Check sheet for the modelled part. Datum: model origin and axes. Units: mm. Face numbers are marked on the shaded views. A direction names the side the tool comes from. Coordinates: 2 decimals unless noted, no trailing zeros. Write each loop counter-clockwise with the first axis right and the second up, starting at its lowest first coordinate (ties: lowest second). Pieces come first, ordered by that corner, then holes. Notation, with made-up numbers: M 87,34 L 146,34 A22 ccw 146,40 Z; hole C -21,-19 d6. An arc over 180 degrees is marked long. Answer as CSV lines item,"result". Start each with the question number.
1) Section check C-C (y = 20.75). Record the cut outline in (x, z).
2) Section check A-A (y = 4.5). Record the cut outline in (x, z).
3) Go/stop test with flat-tipped pins: pin 1 Ø2 at (x, y) = (-15.5, 4) entering from -Z; pin 2 Ø6 at (y, z) = (7.5, 2.5) entering from +X; pin 3 Ø1 at (x, y) = (-15, 4.5) entering from +Z. Record where each tip stops, or that it passes through.
4) Section check D-D (x = -6). Record the cut outline in (y, z).
5) Section check B-B (z = -12). Record the cut outline in (x, y).
6) Access from +Z, -Z, +X, -X, +Y, -Y to the whole of each face (thin tool, end or side, straight path). Record for the marked faces 4, 5, 6 and 7.
7) Material ranges on L1, parallel to Z at x = -6.5, y = 10.25; L2, parallel to Z at x = 15, y = 2, recorded low to high. Write a range as [from, to].
8) Draft check along X on the marked faces 1, 2 and 3. Enter one of: +X half, -X half, draft (parallel to the pull), parting line (faces both ways), or undercut.
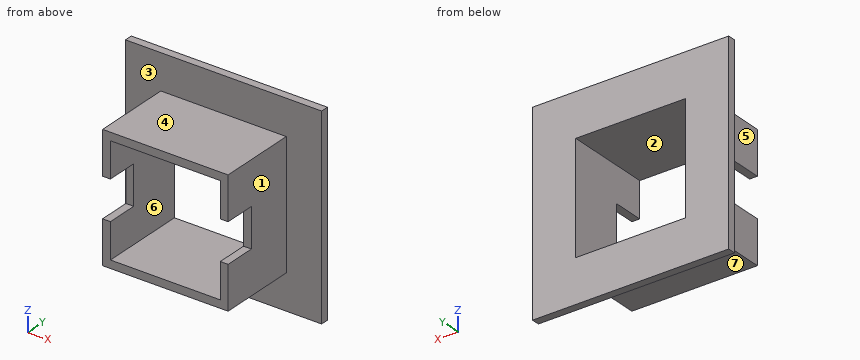
from build123d import *

# Parameters (mm, degrees)
SKETCH1_W           = 32
SKETCH1_H           = 32
SKETCH1_W_2         = 28
SKETCH1_H_2         = 28
BOSS_EXTRUDE1_DEPTH = 20
SKETCH2_W           = 10
SKETCH2_H           = 8
CUT_EXTRUDE1_DEPTH  = 33
SKETCH3_W           = 50
SKETCH3_H           = 50
SKETCH3_W_2         = 28
SKETCH3_H_2         = 28
BOSS_EXTRUDE2_DEPTH = 2


with BuildPart() as part:
    # Sketch1 → Boss-Extrude1 (new body)
    with BuildSketch(Plane(origin=(0, 0, 0), x_dir=(1, 0, 0), z_dir=(0, 1, 0))):
        Rectangle(SKETCH1_W, SKETCH1_H)
        Rectangle(SKETCH1_W_2, SKETCH1_H_2, mode=Mode.SUBTRACT)
    extrude(amount=BOSS_EXTRUDE1_DEPTH)

    # Sketch2 → Cut-Extrude1 (cut, through all)
    with BuildSketch(Plane(origin=(16, 0, 0), x_dir=(0, 0, -1), z_dir=(1, 0, 0))):
        with Locations((0, 4)):
            Rectangle(SKETCH2_W, SKETCH2_H)
    extrude(amount=-CUT_EXTRUDE1_DEPTH, mode=Mode.SUBTRACT)

    # Sketch3 → Boss-Extrude2 (add)
    with BuildSketch(Plane(origin=(0, 20, 0), x_dir=(1, 0, 0), z_dir=(0, 1, 0))):
        Rectangle(SKETCH3_W, SKETCH3_H)
        Rectangle(SKETCH3_W_2, SKETCH3_H_2, mode=Mode.SUBTRACT)
    extrude(amount=BOSS_EXTRUDE2_DEPTH)


solid = part.part
Results found:
1,outline,"M -25,-25 L 25,-25 L 25,25 L -25,25 Z; hole M -14,-14 L 14,-14 L 14,14 L -14,14 Z"
2,outline,"M -16,-16 L 16,-16 L 16,-5 L 14,-5 L 14,-14 L -14,-14 L -14,-5 L -16,-5 Z; M -16,5 L -14,5 L -14,14 L 14,14 L 14,5 L 16,5 L 16,16 L -16,16 Z"
3,pin 1,"stops at z = -16"
3,pin 2,"stops at x = 16"
3,pin 3,"stops at z = 16"
4,outline,"M 0,-16 L 20,-16 L 20,-25 L 22,-25 L 22,-14 L 0,-14 Z; M 0,14 L 22,14 L 22,25 L 20,25 L 20,16 L 0,16 Z"
5,outline,"M -25,20 L -16,20 L -16,0 L -14,0 L -14,22 L -25,22 Z; M 14,0 L 16,0 L 16,20 L 25,20 L 25,22 L 14,22 Z"
6,face 4,"+Z, +X, -X, -Y"
6,face 5,"+Z, -Z, -X, -Y"
6,face 6,"+Y, -Y"
6,face 7,"-Z, +X, -X, -Y"
7,L1,"z = [-16, -14], [14, 16]"
7,L2,"z = [-16, -5], [5, 16]"
8,face 1,"+X half"
8,face 2,"undercut"
8,face 3,"draft"
